Source: CAD feature listing. Evaluate the final solid. Frame: model axes, mm. A direction names the side the tool comes from. Give positions to 0.01 mm unless a question says otherwise; leave off trailing zeros. Loops run counter-clockwise (first coordinate to the right, second up) from the corner with the lowest first, then second, coordinate; pieces in that order, holes last.
Autodesk Inventor part; units mm, degrees
ref_plane "YZ Plane" through (0, 0, 0) normal (1, 0, 0) x (0, 1, 0)
ref_plane "XZ Plane" through (0, 0, 0) normal (0, 1, 0) x (-1, 0, 0)
ref_plane "XY Plane" through (0, 0, 0) normal (0, 0, 1) x (1, 0, 0)
sketch "Sketch1" plane through (0, 0, 0) normal (0, 1, 0) x (-1, 0, 0)
  line L0 (10, 67.88) -> (-10, 67.88)
  line L1 (-10, 67.88) -> (-10, -10)
  line L2 (-10, -10) -> (10, -10)
  line L3 (10, -10) -> (10, 67.88)
  point P0 (0, 0)
  dimension "d0" = 20
  dimension "d1" = 77.88
extrude "Extrusion1" add sketch "Sketch1" along normal blind 2
sketch "Sketch2" plane through (0, 2, 0) normal (0, 1, 0) x (1, 0, 0)
  line L0 (-10, -67.88) -> (10, -67.88)
  line L1 (0, -67.88) -> (-6.35, -67.88)
  line L2 (-6.35, -56.98) -> (6.35, -56.98)
  line L3 (6.35, -67.88) -> (0, -67.88)
  line L4 (10, 10) -> (-10, 10)
  line L5 (-6.35, -0.9) -> (6.35, -0.9)
  line L6 (-6.35, 10) -> (6.35, 10)
  line L7 (-6.35, -67.88) -> (-10, -67.88)
  line L8 (-10, 10) -> (-10, -67.88)
  line L9 (-10, -56.98) -> (-6.35, -56.98)
  line L10 (6.35, -67.88) -> (10, -67.88)
  line L11 (10, -67.88) -> (10, 10)
  line L12 (10, -56.98) -> (6.35, -56.98)
  line L13 (6.35, -0.9) -> (10, -0.9)
  line L14 (10, 10) -> (6.35, 10)
  line L15 (10, -0.9) -> (10, 10)
  line L16 (10, -67.88) -> (10, -56.98)
  line L17 (-10, -67.88) -> (-10, -56.98)
  line L18 (-6.35, -0.9) -> (-10, -0.9)
  line L19 (-10, -0.9) -> (-10, 10)
  line L20 (-10, 10) -> (-6.35, 10)
  point P0 (0, 0)
  dimension "d4" = 6.35
  dimension "d5" = 10.9
  dimension "d6" = 12.7
  dimension "d7" = 10.9
extrude "Extrusion2" add sketch "Sketch2" along normal blind 48.3354 contours L8 L9 L2 L12 L11 L0 | L8 L4 L11 L13 L5 L18
sketch "Sketch9" plane through (-10, 0, 67.88) normal (0, 0, 1) x (1, 0, 0)
  arc A0 (15.084, 42.3223) -> (4.684, 42.3223) centre (9.884, 42.3223) ccw
  line L0 (15.084, 35.9247) -> (15.084, 42.3223)
  line L1 (4.684, 41.1247) -> (4.684, 42.3223)
  arc A1 (15.084, 42.3223) -> (4.684, 42.3223) centre (9.884, 42.3223) ccw
  line L2 (4.684, 42.3223) -> (4.684, 35.9247)
  line L3 (9.8827, 20.3222) -> (-0.0013, 20.3222)
  line L4 (-0.0013, 30.726) -> (-0.0013, 20.3222)
  line L5 (4.684, 35.9247) -> (4.684, 30.726)
  line L6 (15.084, 35.9247) -> (15.0853, 25.5254)
  arc A2 (15.084, 35.9247) -> (15.084, 35.9251) centre (9.884, 35.9243) ccw
  line L7 (4.684, 30.726) -> (-0.0013, 30.726)
  arc A3 (9.8827, 20.3222) -> (15.0853, 25.5254) centre (9.8827, 25.5248) ccw
  point P0 (10, 0)
fillet "Fillet4" radius 10 4 edges at (10, 50.3354, 62.43) (-10, 50.3354, 62.43) (-10, 50.3354, -4.55) (10, 50.3354, -4.55)
sketch "Sketch10" plane through (0, 2, 0) normal (0, 1, 0) x (1, 0, 0)
  line L0 (10, -67.88) -> (-10, -67.88)
  line L1 (-10, 10) -> (10, 10)
  line L2 (10, -56.98) -> (10, -0.9)
  line L3 (-10, -0.9) -> (-10, -56.98)
  line L4 (10, -28.94) -> (-10, -28.94)
  circle A0 centre (0, -28.94) radius 2.125
  point P0 (0, 0)
  dimension "d53" = 77.88
  dimension "d54" = 4.25
extrude "Extrusion10" cut sketch "Sketch10" against normal blind 2
extrude "Extrusion11" cut sketch "Sketch9" against normal through all
sketch "Sketch11" plane through (10, 0, 67.88) normal (1, 0, 0) x (0, 0, -1)
  line L0 (0, 0) -> (0, 20.3222)
  line L1 (77.88, 30.726) -> (77.88, 40.3354)
  line L2 (0, 0) -> (77.88, 0)
  line L3 (77.88, 0) -> (77.88, 40.3354)
  line L4 (77.88, 40.3354) -> (0, 40.3354)
  line L5 (0, 40.3354) -> (0, 0)
  point P0 (67.88, 0)
extrude "Extrusion12" add sketch "Sketch11" along normal blind 2
sketch "Sketch12" plane through (12, 0, 67.88) normal (1, 0, 0) x (0, 0, -1)
  line L0 (10.9, 40.3354) -> (0, 40.3354)
  line L1 (77.88, 30.726) -> (77.88, 40.3354)
  line L2 (0, 40.3354) -> (77.88, 40.3354)
  line L3 (77.88, 40.3354) -> (0, 40.3354)
  line L4 (38.94, 40.3354) -> (64.34, 40.3354)
  line L5 (38.94, 40.3354) -> (13.54, 40.3354)
  line L6 (77.88, 0) -> (0, 0)
  line L7 (13.54, 40.3354) -> (64.34, 40.3354)
  line L8 (64.34, 40.3354) -> (64.34, 0)
  line L9 (64.34, 0) -> (13.54, 0)
  line L10 (13.54, 0) -> (13.54, 40.3354)
  line L11 (13.54, 0) -> (31.84, 0)
  line L12 (31.84, 0) -> (31.84, 6)
  arc A0 (33.84, 36.3354) -> (29.84, 36.3354) centre (31.84, 36.3354) ccw
  arc A1 (29.84, 6) -> (33.84, 6) centre (31.84, 6) ccw
  line L13 (29.84, 36.3354) -> (29.84, 6)
  line L14 (33.84, 36.3354) -> (33.84, 6)
  line L15 (31.84, 36.3354) -> (13.54, 36.3354)
  point P0 (67.88, 0)
  dimension "d65" = 25.4
  dimension "d66" = 25.4
  dimension "d67" = 50.8
  dimension "d68" = 18.3
  dimension "d69" = 6
  dimension "d71" = 4
  dimension "d72" = 4
  dimension "d75" = 18.3
extrude "Extrusion13" cut sketch "Sketch12" against normal blind 2 contours A0 L14 A1 L13
properties part number "6 Backet Adjustment 2.0"
(1) Section B-B, the plane z = 28.94. Return the cut outline in (x, y) (1 decimal).
A:
outline: (-10, 0) - (-2.1, 0) - (-2.1, 2) - (-10, 2) - close; (2.1, 0) - (12, 0) - (12, 40.3) - (10, 40.3) - (10, 2) - (2.1, 2) - close
(2) Mould query, pull axis Z, two halves, no side actions, for faces 5 (the cylindrical face through (-6.993, 47.484, -4.474)), 6 (the cylindrical face through (11, 4, 36)), 7 (the flat face through (1, 19, 67.88)). Classes: pulls with the +Z half, pulls with the -Z half, needs draft (parallel to the pull), parting line crosses it, or undercut.
A:
face 5: needs draft
face 6: undercut
face 7: pulls with the +Z half
(3) Section A-A, the plane y = 17. Return the cut outline in (x, z).
A:
outline: (-10, -10) - (12, -10) - (12, 34.04) - (10, 34.04) - (10, 0.9) - (-10, 0.9) - close; (-10, 56.98) - (10, 56.98) - (10, 38.04) - (12, 38.04) - (12, 67.88) - (-10, 67.88) - close
(4) Reachability of faces 1 (the flat face through (-5.316, 36, -4)), 2 (the cylindrical face through (11.014, 38.335, 35.996)), 3 (the flat face through (2.4, 2, 29.3)), 4 (the flat face through (-8, 30.726, 63)) from +Z, -Z, +X, -X, +Y, -Y: full face, straight path, thin tool, end or side. Return the list, or none.
A:
face 1: +Z, -Z
face 2: +X, -X
face 3: -X, +Y
face 4: +Z, -Z, -X
(5) Ray query, line 1 along X through (y, z) = (1.45, 28.94) (3 decimals); line 2 along Z through (x, y) = (0, 1.5) (3 decimals); line 3 along Z through (x, y) = (-8.5, 40). Return the intervals inside material, ascending.
A:
line 1: x = -10 to -2.125, 2.125 to 12
line 2: z = -10 to 26.815, 31.065 to 67.88
line 3: z = -10 to 0.9, 56.98 to 67.88
(6) First-contact query: pin 1 (8.5 mm diameter, centred on y = 28.5, z = 63, fed in from -X); pin 2 (6 mm diameter, centred on y = 14.5, z = 24, fed in from -X); pin 3 (5 mm diameter, centred on x = -6.5, z = -6.5, fed in from +Y); pin 4 (5 mm diameter, centred on x = 5.5, z = 9, fed in from +Y). Flat tips, straight axial feed; report the tip coordinate or a pass-through.
A:
pin 1: stops at x = -10
pin 2: stops at x = 10
pin 3: stops at y = 49.5
pin 4: stops at y = 2
(7) Section C-C, the plane x = 3.25. Return the cut outline in (y, z), then the cut area to 3 significant figures.
A:
outline: (0, -10) - (21.56, -10) - (21.56, 0.9) - (2, 0.9) - (2, 56.98) - (21.56, 56.98) - (21.56, 67.88) - (0, 67.88) - close; (46.29, -10) - (49.79, -10) - (49.79, 0.9) - (46.29, 0.9) - close; (46.29, 56.98) - (49.79, 56.98) - (49.79, 67.88) - (46.29, 67.88) - close
area: 659 mm2
(8) Section D-D, the plane y = 45. Return the cut outline in (x, z).
A:
outline: (-8.85, -10) - (-4.57, -10) - (-4.57, 0.9) - (-8.85, 0.9) - close; (-8.85, 56.98) - (-4.57, 56.98) - (-4.57, 67.88) - (-8.85, 67.88) - close; (4.34, -10) - (8.85, -10) - (8.85, 0.9) - (4.34, 0.9) - close; (4.34, 56.98) - (8.85, 56.98) - (8.85, 67.88) - (4.34, 67.88) - close
